from build123d import *

# Parameters (mm, degrees)
F6_R     = 0.75
F7_DEPTH = 9


with BuildPart() as f1:
    # F0 (on Right) → F1 (revolve)
    with BuildSketch(Plane.YZ):
        Polygon((1.25, 7), (0, 7), (0, 0), (33.25, 0), (33.25, 2.7), (33.5, 3.133013), (33.5, 4.756052), (30, 5.5), (30, 5), (21.5, 5), (21.5, 4.65), (10.9, 4.65), (10.9, 6.5), (2.5, 6.5), (2.5, 4.65), (1.5, 4.65), align=None)
    revolve(axis=Axis((0, -17.104737, 0), (0, -1, 0)))

    # F2 (on Right) → F3 (revolve)
    with BuildSketch(Plane.YZ):
        Polygon((-8.497705, 5.5), (0, 5.5), (0, 7.35), (-6, 7.35), (-6, 7), (-9, 7), (-9, 6.37), align=None)
    revolve(axis=Axis((0, -12.747619, 0), (0, -1, 0)))

    # F4 (on Right) → F5 (revolve)
    with BuildSketch(Plane.YZ):
        Polygon((-10, 0), (0, 0), (0, 5.25), (-1, 5.25), (-1, 4), (-10, 4), align=None)
    revolve(axis=Axis((0, -5, 0), (0, 1, 0)))

    # F6 (on face) → F7 (cut, through all)
    with BuildSketch(Plane.XZ.offset(10)):
        with Locations((-2, 2)):
            Circle(F6_R)
        with Locations((2, 2)):
            Circle(F6_R)
        with Locations((2, -2)):
            Circle(F6_R)
        with Locations((-2, -2)):
            Circle(F6_R)
        with BuildLine():
            ThreePointArc((-0.6, 3.5), (-0.453553, 3.146447), (-0.1, 3))
            Line((-0.1, 3), (0.1, 3))
            ThreePointArc((0.1, 3), (0.453553, 3.146447), (0.6, 3.5))
            Line((0.6, 3.5), (0.6, 4.5))
            Line((0.6, 4.5), (-0.6, 4.5))
            Line((-0.6, 4.5), (-0.6, 3.5))
        make_face()
    extrude(amount=-F7_DEPTH, mode=Mode.SUBTRACT)


solid = f1.part
Read the model definition and answer for the solid it produces. Units are mm, in the model's axes. A direction names the side the tool comes from. Coordinates: 2 decimals unless noted, no trailing zeros. Write each loop counter-clockwise with the first axis right and the second up, starting at its lowest first coordinate (ties: lowest second). Pieces come first, ordered by that corner, then holes. Notation, with made-up numbers: (-27.5, -9.75) -> (18.5, -9.75) arc R28 ccw to (18.5, 16.25) -> close; hole circle Ø10 at (-33, 56). An arc over 180 degrees is marked (long way). Return JSON: item names as keys, results as strings.
(1) Which of the six approach directions +Z, -Z, +X, -X, +Y, -Y give full straight-line access (tool end or side, diameter ignored) to faces 5 (the cylindrical face through (3.955, 6.641, -5.158)), 6 (the flat face through (0, -10, 0)), 7 (the cylindrical face through (-3.92, 1.99, 2.5)), 8 (the cylindrical face through (2.681, -7.521, 6.466))?
Answers below:
{"face 5": "+Y", "face 6": "+Z, -Z, +X, -X, -Y", "face 7": "none", "face 8": "-Y"}
(2) Each of these flat-tipped pins is pushed along its axis until it touches: P1, Ø1.5, axis at y = -2.5, z = -6, coming from the -X side; P2, Ø1.6, axis at x = -1, z = -0.5, coming from the +Y side; P3, Ø1.5, axis at y = 25, z = 1, coming from the +X side. Where does it stop, or does it pass through?
Answers below:
{"P1": "x = -5.14", "P2": "y = 33.25", "P3": "x = 4.99"}
(3) Consider line 1 along X through (y, z) = (-5.75, 0); line 2 along Z through (x, y) = (2, -6.75); line 3 along Z through (x, y) = (2, -5.5). Determine where each line is inside the solid, lowest interval first. Write a range as from..to.
Answers below:
{"line 1": "-7.35..-5.5, -4..4, 5.5..7.35", "line 2": "-6.71..-5.12, -3.46..-2.75, -1.25..1.25, 2.75..3.46, 5.12..6.71", "line 3": "-7.07..-5.12, -3.46..-2.75, -1.25..1.25, 2.75..3.46, 5.12..7.07"}
(4) The part is cut by section C-C on y = 29. Give the vertices of the cut face in (x, z).
Answers below:
{"outline": "circle Ø10 at (0, 0)"}
(5) The part is cut by section B-B on y = 14. Give the vertices of the cut face in (x, z).
Answers below:
{"outline": "circle Ø9.3 at (0, 0)"}
(6) For a pull along Z with two mould halves and no side action, classify faces 1 (the flat face through (-2, -1, -2)), 2 (the flat face through (2, -1, 2)), 3 (the cylindrical face through (-3.92, 16.13, 2.5)), 4 (the flat face through (6, -9, 3)) as pulls with the +Z half, pulls with the -Z half, needs draft (parallel to the pull), parting line crosses it, or undercut.
Answers below:
{"face 1": "undercut", "face 2": "undercut", "face 3": "parting line crosses it", "face 4": "needs draft"}
(7) The part is cut by section A-A on y = -2. Give the vertices of the cut face in (x, z), then the cut area to 3 significant figures.
Answers below:
{"outline": "circle Ø14.7 at (0, 0); (-0.6, 3.5) -> (-0.6, 3.95) arc R4 ccw (long way) to (0.6, 3.95) -> (0.6, 3.5) arc R0.5 cw to (0.1, 3) -> (-0.1, 3) arc R0.5 cw to start; hole circle Ø11 at (0, 0); hole circle Ø1.5 at (-2, -2); hole circle Ø1.5 at (-2, 2); hole circle Ø1.5 at (2, -2); hole circle Ø1.5 at (2, 2)", "area": "117 mm^2"}
